from build123d import *

# Parameters (mm, degrees)
SKETCH_2_R      = 3.5
SKETCH_2_R_2    = 1.5
EXTRUDE_1_DEPTH = 3
FILLET_1_R      = 14
SKETCH_3_W      = 5
SKETCH_3_H      = 3
EXTRUDE_2_DEPTH = 3
EXTRUDE_4_DEPTH = 3


with BuildPart() as part:
    # 草图2 → 凸台-拉伸1 (new body)
    # profile 1 of 3: a face of its own
    with BuildSketch(Plane(origin=(0, 0, 0), x_dir=(1, 0, 0), z_dir=(0, 1, 0))):
        with Locations((-16, 0)):
            Circle(SKETCH_2_R)
        with Locations(Location((-16, 0, 0), (0, 0, 270))):
            Circle(SKETCH_2_R_2, mode=Mode.SUBTRACT)
    # profile 2 of 3: a face of its own
    with BuildSketch(Plane(origin=(0, 0, 0), x_dir=(1, 0, 0), z_dir=(0, 1, 0))):
        Circle(SKETCH_2_R)
        with Locations(Location((0, 0, 0), (0, 0, 270))):
            Circle(SKETCH_2_R_2, mode=Mode.SUBTRACT)
    # profile 3 of 3: a face of its own
    with BuildSketch(Plane(origin=(0, 0, 0), x_dir=(1, 0, 0), z_dir=(0, 1, 0))):
        with BuildLine():
            Line((-3.16227766, 1.5), (-12.83772234, 1.5))
            ThreePointArc((-12.83772234, 1.5), (-12.585474278, 0.768774411), (-12.5, 0))
            ThreePointArc((-12.5, 0), (-17.197070502, -3.288924173), (-18.681155551, 2.249756634))
            Line((-18.681155551, 2.249756634), (-29.392987934, -10.516108092))
            Line((-29.392987934, -10.516108092), (0.110005112, -5.313934406))
            Line((0.110005112, -5.313934406), (2.681155551, -2.249756634))
            ThreePointArc((2.681155551, -2.249756634), (-1.890248218, -2.94566829), (-3.16227766, 1.5))
        make_face()
    extrude(amount=EXTRUDE_1_DEPTH)

    # 圆角1
    # the kernel refuses this fillet: 14 mm, written as the material it adds along each edge
    with BuildSketch(Plane(origin=(-3.16227766, 0, -1.5), x_dir=(-1, 0, 0), z_dir=(0, 1, 0))) as fillet_1_piece_1:
        with BuildLine():
            CenterArc((4.961760744, -14), FILLET_1_R, 90, 27.660449899)
            ThreePointArc((-1.537469979, -1.6), (-0.638580667, -0.925067728), (0, 0))
            Line((0, 0), (4.961760744, 0))
        make_face()
    extrude(amount=3)
    with BuildSketch(Plane(origin=(-12.83772234, 0, -1.5), x_dir=(-0.6928764936482941, 0, -0.721056283898591), z_dir=(0, 1, 0))) as fillet_1_piece_2:
        with BuildLine():
            CenterArc((6.656900588, -13.277979675), FILLET_1_R, 108.481308288, 27.660449899)
            Line((-3.437887387, -3.577708764), (0, 0))
            ThreePointArc((0, 0), (1.109483431, -0.180505081), (2.218966863, 0))
        make_face()
    extrude(amount=3)

    # 草图3 → 凸台-拉伸2 (add)
    with BuildSketch(Plane(origin=(0.912053364, 0, 5.17251166), x_dir=(0.9848077530122087, 0, -0.17364817766692722), z_dir=(0.17364817766692722, 0, 0.9848077530122087))):
        with Locations((-21.814421139, 1.5)):
            Rectangle(SKETCH_3_W, SKETCH_3_H)
        with Locations((-6.814421139, 1.5)):
            Rectangle(SKETCH_3_W, SKETCH_3_H)
    extrude(amount=EXTRUDE_2_DEPTH)

    # 草图5 → 凸台-拉伸4 (add)
    with BuildSketch(Plane.XZ):
        with BuildLine():
            ThreePointArc((-1.118033989, -1), (0, -1.5), (1.118033989, -1))
            Line((1.118033989, -1), (-1.118033989, -1))
        make_face()
        with BuildLine():
            ThreePointArc((-17.118033989, -1), (-16, -1.5), (-14.881966011, -1))
            Line((-14.881966011, -1), (-17.118033989, -1))
        make_face()
    extrude(amount=-EXTRUDE_4_DEPTH)


solid = part.part
Verification items for the finished model (mm, model axes). A direction names the side the tool comes from. Give positions to 0.01 mm unless a question says otherwise; leave off trailing zeros. Loops run counter-clockwise (first coordinate to the right, second up) from the corner with the lowest first, then second, coordinate; pieces in that order, holes last.
1. Material ranges on probe 1 along X at (y, z) = (1.25, 0); probe 2 along X at (y, z) = (2.25, -0.5); probe 3 along Z at (x, y) = (0, 1.5), recorded low to high.
Derived:
probe 1: x = -20.57 to -17.5, -14.5 to -1.5, 1.5 to 3.5
probe 2: x = -20.15 to -17.41, -14.59 to -1.41, 1.41 to 3.46
probe 3: z = -3.5 to -1, 1.5 to 5.33
2. Cross-section at B-B on y = 1. Record the cut outline in (x, z), and give its area (3 significant figures).
Derived:
outline: (-29.39, 10.52) - (-18.68, -2.25) arc R3.5 ccw to (-14.38, -3.1) arc R14 cw to (-8, -1.5) arc R14 cw to (-1.62, -3.1) arc R3.5 ccw to (2.68, 2.25) - (0.11, 5.31) - (-3.34, 5.92) - (-2.82, 8.88) - (-7.74, 9.74) - (-8.26, 6.79) - (-18.11, 8.53) - (-17.59, 11.48) - (-22.51, 12.35) - (-23.03, 9.39) - close; hole (-17.12, -1) - (-14.88, -1) arc R1.5 ccw (long way) to start; hole (-1.12, -1) - (1.12, -1) arc R1.5 ccw (long way) to start
area: 272 mm2
3. Go/stop test with flat-tipped pins: P1, Ø1.1, axis at x = 0.5, y = 1.5, coming from the +Z side; P2, Ø1.5, axis at x = -10, y = 1, coming from the -Z side; P3, Ø0.7, axis at x = -15.5, y = 2, coming from the +Z side. Record where each tip stops, or that it passes through.
Derived:
P1: stops at z = 5.34
P2: stops at z = -1.8
P3: stops at z = 8.13
4. Cross-section at C-C on x = -16. Record the cut outline in (y, z).
Derived:
outline: (0, -3.5) - (3, -3.5) - (3, -1) - (0, -1) - close; (0, 1.5) - (3, 1.5) - (3, 8.15) - (0, 8.15) - close
5. Release check for a two-part mould opening along Z. For faces 4 (the cylindrical face through (-16.65, 1.48, -3.44)), 5 (the flat face through (-22.776, 1.479, 10.851)), 6 (the flat face through (0, 1, -1)) record: +Z half, -Z half, draft (parallel to the pull), parting line (faces both ways), or undercut.
Derived:
face 4: -Z half
face 5: +Z half
face 6: undercut
6. Cross-section at A-A on z = 7.75. Record the cut outline in (x, y), and give its area (3 significant figures).
Derived:
outline: (-27.07, 0) - (-13.71, 0) - (-13.71, 3) - (-27.07, 3) - close; (-8.09, 0) - (-3.01, 0) - (-3.01, 3) - (-8.09, 3) - close
area: 55.3 mm2
7. Cross-section at D-D on z = 0.5. Record the cut outline in (x, y), and give its area (3 significant figures).
Derived:
outline: (-20.99, 0) - (-17.41, 0) - (-17.41, 3) - (-20.99, 3) - close; (-14.59, 0) - (-1.41, 0) - (-1.41, 3) - (-14.59, 3) - close; (1.41, 0) - (3.46, 0) - (3.46, 3) - (1.41, 3) - close
area: 56.4 mm2
8. Tool access check on faces 1 (the flat face through (-17.852, 1.479, 9.983)), 2 (the flat face through (-8.004, 1.479, 8.246)), 3 (the cylindrical face through (-11.328, 1.479, -1.932)). Record the directions out of +Z, -Z, +X, -X, +Y, -Y that give a thin tool (end or side, any length) a straight path to the whole face; none if there is none.
Derived:
face 1: +Y, -Y
face 2: +Z, +Y, -Y
face 3: -Z, +Y, -Y
